Check sheet for the modelled part. Datum: model origin and axes. Units: mm. Round coordinates to 2 decimals unless told otherwise and drop trailing zeros. Write each loop counter-clockwise with the first axis right and the second up, starting at its lowest first coordinate (ties: lowest second). Pieces come first, ordered by that corner, then holes. Notation, with made-up numbers: (54, -35.5) - (62, -35.5) arc R13 cw to (62, -11.5) - close; hole circle Ø3 at (8, -9). An arc over 180 degrees is marked (long way). Answer as a JSON object with one key per item and string values. Group by question number.
Item 1: Sectioned sample at C-C on x = 12.7. Record the boundary of the cut face in (y, z), plus the area to 3 significant figures.
Item 2: Release check for a two-part mould opening along Y. For faces 1 (the flat face through (63, 64, 1.588)), 2 (the flat face through (64, 127, 0)), 3 (the cylindrical face through (10.72, 87.39, -0.02)) record: pulls with the +Y half, pulls with the -Y half, needs draft (parallel to the pull), parting line crosses it, or undercut.
Item 3: Thickness scan on line 1 (Y direction, x = 12.7, z = -0.7); line 2 (Y direction, x = 63.5, z = 0.6); line 3 (Y direction, x = 13.5, z = 0.45). Record the ranges inside material, lowest first.
Item 4: Sectioned sample at A-A on y = 38.1. Record the boundary of the cut face in (x, z), plus the area to 3 significant figures.
```python
from build123d import *

# Parameters (mm, degrees)
SKETCH1_R           = 2.4892
BOSS_EXTRUDE1_DEPTH = 1.5875


with BuildPart() as part:
    # Sketch1 → Boss-Extrude1 (new, symmetric)
    with BuildSketch(Plane.XY):
        Polygon((0, 127), (0, 0), (127, 0), (127, 25.4), (127, 127), align=None)
        with Locations((114.3, 12.7)):
            Circle(SKETCH1_R, mode=Mode.SUBTRACT)
        with Locations((88.9, 12.7)):
            Circle(SKETCH1_R, mode=Mode.SUBTRACT)
        with Locations((63.5, 12.7)):
            Circle(SKETCH1_R, mode=Mode.SUBTRACT)
        with Locations((38.1, 12.7)):
            Circle(SKETCH1_R, mode=Mode.SUBTRACT)
        with Locations((12.7, 12.7)):
            Circle(SKETCH1_R, mode=Mode.SUBTRACT)
        with Locations((12.7, 38.1)):
            Circle(SKETCH1_R, mode=Mode.SUBTRACT)
        with Locations((12.7, 63.5)):
            Circle(SKETCH1_R, mode=Mode.SUBTRACT)
        with Locations((12.7, 88.9)):
            Circle(SKETCH1_R, mode=Mode.SUBTRACT)
        with Locations((12.7, 114.3)):
            Circle(SKETCH1_R, mode=Mode.SUBTRACT)
    extrude(amount=BOSS_EXTRUDE1_DEPTH, both=True)


solid = part.part
```
Completed:
{
 "1": {"outline": "(0, -1.59) - (10.21, -1.59) - (10.21, 1.59) - (0, 1.59) - close; (15.19, -1.59) - (35.61, -1.59) - (35.61, 1.59) - (15.19, 1.59) - close; (40.59, -1.59) - (61.01, -1.59) - (61.01, 1.59) - (40.59, 1.59) - close; (65.99, -1.59) - (86.41, -1.59) - (86.41, 1.59) - (65.99, 1.59) - close; (91.39, -1.59) - (111.81, -1.59) - (111.81, 1.59) - (91.39, 1.59) - close; (116.79, -1.59) - (127, -1.59) - (127, 1.59) - (116.79, 1.59) - close", "area": "324 mm²"},
 "2": {"face 1": "needs draft", "face 2": "pulls with the +Y half", "face 3": "undercut"},
 "3": {"line 1": "0 to 10.21, 15.19 to 35.61, 40.59 to 61.01, 65.99 to 86.41, 91.39 to 111.81, 116.79 to 127", "line 2": "0 to 10.21, 15.19 to 127", "line 3": "0 to 10.34, 15.06 to 35.74, 40.46 to 61.14, 65.86 to 86.54, 91.26 to 111.94, 116.66 to 127"},
 "4": {"outline": "(0, -1.59) - (10.21, -1.59) - (10.21, 1.59) - (0, 1.59) - close; (15.19, -1.59) - (127, -1.59) - (127, 1.59) - (15.19, 1.59) - close", "area": "387 mm²"}
}
